The listing builds one solid part. Answer for the finished solid, in the listing's coordinates (mm). Face numbers are marked on the shaded views. Round coordinates to 2 decimals unless told otherwise and drop trailing zeros. Order: outer loops, then holes, each group sorted by start corner. A loop starts at its lowest first (then second) coordinate and runs counter-clockwise, first axis right, second up. Notation, with made-up numbers: M 88.5,11 L 117.5,11 A36 ccw 117.5,46 Z; hole C -37,-21.5 d4. An arc over 180 degrees is marked long. Put each result on its own line as item: value. Start each with the question number.
1. The mould has two halves that part along Z. Classify the marked faces 1, 2 and 3: +Z half, -Z half, draft (parallel to the pull), parting line (faces both ways), or undercut.
2. The part is cut by section B-B (z = 0). Give the vertices of the cut face in (x, y), then the cut area to 4 significant figures.
3. The part is cut by section D-D (y = 18.5). Give the vertices of the cut face in (x, z), then the cut area to 3 significant figures.
4. The part is cut by section A-A (x = 0). Give the vertices of the cut face in (y, z), then the cut area to 3 significant figures.
5. Each of these flat-tipped pins is pushed along its axis until it touches: pin 1 Ø2.5 at (x, y) = (0, 9) entering from -Z; pin 2 Ø3 at (y, z) = (10, 13) entering from +X; pin 3 Ø6 at (x, z) = (7, 16) entering from -Y. Where does it stop, or does it pass through?
6. Consider line 1 (X direction, y = 26, z = 0); line 2 (X direction, y = 32, z = 17.5); line 3 (Z direction, x = 0, y = 32.25). Determine where each line is inside the solid, lowest interval first.
7. The part is cut by section C-C (z = 16). Give the vertices of the cut face in (x, y), then the cut area to 3 significant figures.
from build123d import *

# Parameters (mm, degrees)
SKETCH1_R           = 12.5
SKETCH1_R_2         = 5
BOSS_EXTRUDE1_DEPTH = 15
SKETCH2_R           = 41
SKETCH2_R_2         = 5
BOSS_EXTRUDE2_DEPTH = 20
SKETCH3_R           = 3
CUT_EXTRUDE1_DEPTH  = 36
BOSS_EXTRUDE3_DEPTH = 35
SKETCH5_R           = 1.5
CUT_EXTRUDE2_DEPTH  = 37.85
SKETCH6_R           = 41
SKETCH6_R_2         = 12.5
CUT_EXTRUDE3_DEPTH  = 10


with BuildPart() as part:
    # Sketch1 → Boss-Extrude1 (new body)
    with BuildSketch(Plane(origin=(0, 0, 0), x_dir=(1, 0, 0), z_dir=(0, 1, 0))):
        Circle(SKETCH1_R)
        Circle(SKETCH1_R_2, mode=Mode.SUBTRACT)
    extrude(amount=BOSS_EXTRUDE1_DEPTH)

    # Sketch2 → Boss-Extrude2 (add)
    with BuildSketch(Plane(origin=(0, 15, 0), x_dir=(1, 0, 0), z_dir=(0, 1, 0))):
        Circle(SKETCH2_R)
        Circle(SKETCH2_R_2, mode=Mode.SUBTRACT)
    extrude(amount=BOSS_EXTRUDE2_DEPTH)

    # Sketch3 → Cut-Extrude1 (cut, through all)
    with BuildSketch(Plane(origin=(0, 35, 0), x_dir=(1, 0, 0), z_dir=(0, 1, 0))):
        with Locations((0, 35)):
            Circle(SKETCH3_R)
        with Locations((30.310889132, 17.5)):
            Circle(SKETCH3_R)
        with Locations((30.310889132, -17.5)):
            Circle(SKETCH3_R)
        with Locations((0, -35)):
            Circle(SKETCH3_R)
        with Locations((-30.310889132, -17.5)):
            Circle(SKETCH3_R)
        with Locations((-30.310889132, 17.5)):
            Circle(SKETCH3_R)
    extrude(amount=-CUT_EXTRUDE1_DEPTH, mode=Mode.SUBTRACT)

    # Sketch4 → Boss-Extrude3 (add)
    with BuildSketch(Plane.XZ):
        with BuildLine():
            ThreePointArc((3.067854181, 4.15), (0, 5.160836103), (-3.067854181, 4.15))
            Line((-3.067854181, 4.15), (3.067854181, 4.15))
        make_face()
    extrude(amount=-BOSS_EXTRUDE3_DEPTH)

    # Sketch5 → Cut-Extrude2 (cut, through all)
    with BuildSketch(Plane(origin=(0, 0, 4.15), x_dir=(-1, 0, 0), z_dir=(0, 0, -1))):
        with Locations((0, 9)):
            Circle(SKETCH5_R)
    extrude(amount=-CUT_EXTRUDE2_DEPTH, mode=Mode.SUBTRACT)

    # Sketch6 → Cut-Extrude3 (cut)
    with BuildSketch(Plane.XZ.offset(-15)):
        Circle(SKETCH6_R)
        Circle(SKETCH6_R_2, mode=Mode.SUBTRACT)
    extrude(amount=-CUT_EXTRUDE3_DEPTH, mode=Mode.SUBTRACT)


solid = part.part
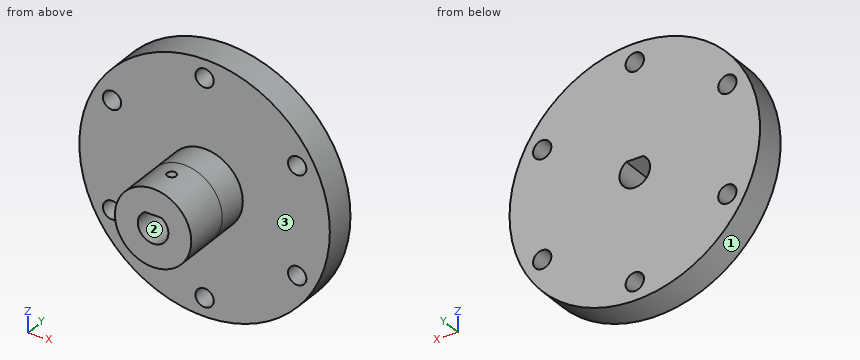
Resolved:
1. face 1: parting line
1. face 2: undercut
1. face 3: draft
2. outline: M -41,25 L -12.5,25 L -12.5,0 L -5,0 L -5,35 L -41,35 Z; M 5,0 L 12.5,0 L 12.5,25 L 41,25 L 41,35 L 5,35 Z
2. area: 1,095 mm2
3. outline: C 0,0 d25; hole M -2.79,4.15 A5 ccw long 2.79,4.15 Z
3. area: 416 mm2
4. outline: M 0,-12.5 L 25,-12.5 L 25,-32 L 35,-32 L 35,-5 L 0,-5 Z; M 0,4.15 L 7.5,4.15 L 7.5,12.5 L 0,12.5 Z; M 10.5,4.15 L 35,4.15 L 35,32 L 25,32 L 25,12.5 L 10.5,12.5 Z; M 25,-41 L 35,-41 L 35,-38 L 25,-38 Z; M 25,38 L 35,38 L 35,41 L 25,41 Z
4. area: 980 mm2
5. pin 1: z = -12.5
5. pin 2: x = 4.9
5. pin 3: y = 25
6. line 1: -41 to -5, 5 to 41
6. line 2: -37.08 to -33.31, -27.31 to 27.31, 33.31 to 37.08
6. line 3: -41 to -38, -32 to -5, 4.15 to 32, 38 to 41
7. outline: M -37.75,25 L -32.91,25 L -32.91,35 L -37.75,35 Z; M -27.71,25 L 27.71,25 L 27.71,35 L -27.71,35 Z; M 32.91,25 L 37.75,25 L 37.75,35 L 32.91,35 Z
7. area: 651 mm2
